```python
from build123d import *

# Parameters (mm, degrees)
SKETCH1_W                   = 203.2
SKETCH1_H                   = 44.4627
CHAMFER1_SIZE               = 1.524
CUT_EXTRUDE2_START          = -88.9254
SKETCH2_W                   = 44.45
SKETCH2_H                   = 38.1
CUT_EXTRUDE2_DEPTH          = 177.8508
FILLET1_R                   = 6.35
CUT_EXTRUDE4_START          = 31.7627
SKETCH3_W                   = 47.752
SKETCH3_H                   = 44.45
CUT_EXTRUDE4_DEPTH          = 88.9254
FILLET2_R                   = 6.35
CUT_EXTRUDE6_START          = -101.6
SKETCH4_R                   = 18.0578125
CUT_EXTRUDE6_DEPTH          = 63.5
CUT_EXTRUDE8_START          = 101.6
SKETCH5_R                   = 6.7437
CUT_EXTRUDE8_DEPTH          = 95.25
CUT_EXTRUDE10_START         = 101.6
SKETCH6_R                   = 10.3124
CUT_EXTRUDE10_DEPTH         = 31.75
F_3_8_16_TAPPED_HOLE2_D     = 7.9375
F_3_8_16_TAPPED_HOLE2_DEPTH = 22.352
F_3_8_16_TAPPED_HOLE2_TIP   = 2.384665582


with BuildPart() as part:
    # Sketch1 → Revolve1 (revolve)
    with BuildSketch(Plane(origin=(0, 0, 0), x_dir=(1, 0, 0), z_dir=(0, 1, 0)), mode=Mode.PRIVATE) as revolve1_sk:
        with Locations((0, 22.23135)):
            Rectangle(SKETCH1_W, SKETCH1_H)
    revolve(revolve1_sk.sketch.rotate(Axis((-127, 0, 0), (1, 0, 0)), 180), axis=Axis((-127, 0, 0), (1, 0, 0)))

    # Chamfer1
    chamfer1_edges = [part.edges().sort_by_distance(p)[0] for p in [
        (101.6, 0, -44.4627),
        (-101.6, 0, -44.4627),
    ]]
    chamfer(chamfer1_edges, length=CHAMFER1_SIZE)

    # Sketch2 → Cut-Extrude2 (cut)
    with BuildSketch(Plane(origin=(0, 0, 0), x_dir=(1, 0, 0), z_dir=(0, 1, 0)).offset(CUT_EXTRUDE2_START)):
        with Locations((-9.525, 0)):
            Rectangle(SKETCH2_W, SKETCH2_H)
    extrude(amount=CUT_EXTRUDE2_DEPTH, mode=Mode.SUBTRACT)

    # Fillet1
    fillet1_edges = [part.edges().sort_by_distance(p)[0] for p in [
        (-31.75, 0, -19.05),
        (-31.75, 0, 19.05),
        (12.7, 0, 19.05),
        (12.7, 0, -19.05),
    ]]
    fillet(fillet1_edges, radius=FILLET1_R)

    # Sketch3 → Cut-Extrude4 (cut)
    with BuildSketch(Plane(origin=(0, 0, 0), x_dir=(1, 0, 0), z_dir=(0, 1, 0)).offset(CUT_EXTRUDE4_START)):
        with Locations((-9.652, 0)):
            Rectangle(SKETCH3_W, SKETCH3_H)
    extrude(amount=CUT_EXTRUDE4_DEPTH, mode=Mode.SUBTRACT)

    # Fillet2
    fillet2_edges = [part.edges().sort_by_distance(p)[0] for p in [
        (-33.528, 35.136096599, -22.225),
        (-33.528, 35.136096599, 22.225),
        (14.224, 35.136096599, 22.225),
        (14.224, 35.136096599, -22.225),
    ]]
    fillet(fillet2_edges, radius=FILLET2_R)

    # Sketch4 → Cut-Extrude6 (cut)
    with BuildSketch(Plane(origin=(0, 0, 0), x_dir=(0, 0, -1), z_dir=(1, 0, 0)).offset(CUT_EXTRUDE6_START)):
        Circle(SKETCH4_R)
    extrude(amount=CUT_EXTRUDE6_DEPTH, mode=Mode.SUBTRACT)

    # Sketch5 → Cut-Extrude8 (cut)
    with BuildSketch(Plane(origin=(0, 0, 0), x_dir=(0, 0, -1), z_dir=(1, 0, 0)).offset(CUT_EXTRUDE8_START)):
        Circle(SKETCH5_R)
    extrude(amount=-CUT_EXTRUDE8_DEPTH, mode=Mode.SUBTRACT)

    # Sketch6 → Cut-Extrude10 (cut)
    with BuildSketch(Plane(origin=(0, 0, 0), x_dir=(0, 0, -1), z_dir=(1, 0, 0)).offset(CUT_EXTRUDE10_START)):
        Circle(SKETCH6_R)
    extrude(amount=-CUT_EXTRUDE10_DEPTH, mode=Mode.SUBTRACT)

    # 3/8-16 Tapped Hole2
    with Locations(Plane(origin=(101.6, 0, 0), x_dir=(0, 0, -1), z_dir=(1, 0, 0))):
        with Locations((-22.4536, -22.4536), (22.4536, -22.4536), (-22.4536, 22.4536), (22.4536, 22.4536)):
            Hole(F_3_8_16_TAPPED_HOLE2_D / 2, depth=F_3_8_16_TAPPED_HOLE2_DEPTH)
            with Locations((0, 0, -(F_3_8_16_TAPPED_HOLE2_DEPTH + F_3_8_16_TAPPED_HOLE2_TIP / 2))):  # 118° drill point
                Cone(0, F_3_8_16_TAPPED_HOLE2_D / 2, F_3_8_16_TAPPED_HOLE2_TIP, mode=Mode.SUBTRACT)


solid = part.part
```
Work out the finished part from the listing and answer in its coordinate system (mm). A direction names the side the tool comes from. Give positions to 0.01 mm unless a question says otherwise; leave off trailing zeros. Loops run counter-clockwise (first coordinate to the right, second up) from the corner with the lowest first, then second, coordinate; pieces in that order, holes last. Notation, with made-up numbers: (87.5, -9.5) - (94.5, -9.5) arc R28 cw to (94.5, 24.5) - close; hole circle Ø1 at (-10, -38). An arc over 180 degrees is marked (long way). One line per question, with ' | ' between items.
(1) Each of these flat-tipped pins is pushed along its axis until it touches: pin 1 Ø6 at (x, y) = (-32, -32.5) entering from +Z; pin 2 Ø7.5 at (x, y) = (-8, 33.5) entering from -Z; pin 3 Ø4 at (x, z) = (77, 27.5) entering from +Y. Where does it stop, or does it pass through?
Recorded:
pin 1: stops at z = 33.27 | pin 2: stops at z = -33.04 | pin 3: stops at y = 36.42
(2) The part is cut by section C-C (y = 0). Write down the section's boundary in (x, z).
Recorded:
outline: (-101.6, -42.94) - (-100.08, -44.46) - (100.08, -44.46) - (101.6, -42.94) - (101.6, -10.31) - (69.85, -10.31) - (69.85, -6.74) - (12.7, -6.74) - (12.7, -12.7) arc R6.35 cw to (6.35, -19.05) - (-25.4, -19.05) arc R6.35 cw to (-31.75, -12.7) - (-31.75, 12.7) arc R6.35 cw to (-25.4, 19.05) - (6.35, 19.05) arc R6.35 cw to (12.7, 12.7) - (12.7, 6.74) - (69.85, 6.74) - (69.85, 10.31) - (101.6, 10.31) - (101.6, 42.94) - (100.08, 44.46) - (-100.08, 44.46) - (-101.6, 42.94) - (-101.6, 18.06) - (-38.1, 18.06) - (-38.1, -18.06) - (-101.6, -18.06) - close
(3) The part is cut by section B-B (x = 54). Write down the section's boundary in (y, z).
Recorded:
outline: circle Ø88.93 at (0, 0); hole circle Ø13.49 at (0, 0)
(4) Straight lines are drawn through the part: probe 1 along Z at (x, y) = (-71.5, -1); probe 2 along Y at (x, z) = (-61.5, 0); probe 3 along X at (y, z) = (3, -7). For each, find the intervals that lie inside material, in ascending order.
Recorded:
probe 1: z = -44.45 to -18.03, 18.03 to 44.45 | probe 2: y = -44.46 to -18.06, 18.06 to 44.46 | probe 3: x = -38.1 to -31.75, 12.7 to 69.85
(5) The part is cut by section A-A (z = 0). Write down the section's boundary in (x, y), then the cut area to 3 significant figures.
Recorded:
outline: (-101.6, -42.94) - (-100.08, -44.46) - (-31.75, -44.46) - (-31.75, 31.76) - (-33.53, 31.76) - (-33.53, 44.46) - (-100.08, 44.46) - (-101.6, 42.94) - (-101.6, 18.06) - (-38.1, 18.06) - (-38.1, -18.06) - (-101.6, -18.06) - close; (12.7, -44.46) - (100.08, -44.46) - (101.6, -42.94) - (101.6, -10.31) - (69.85, -10.31) - (69.85, -6.74) - (12.7, -6.74) - close; (12.7, 6.74) - (69.85, 6.74) - (69.85, 10.31) - (101.6, 10.31) - (101.6, 42.94) - (100.08, 44.46) - (14.22, 44.46) - (14.22, 31.76) - (12.7, 31.76) - close | area: 10,400 mm²
(6) A tool of negligible diameter and unlimited length cuts with its end or side. For faces 4 (the face through (12.7, -7, 0)), 5 (the face through (85.95, 8.7, -5.54)), 6 (the face through (-70.29, -17.63, 3.91)), from which of +Z, -Z, +X, -X, +Y, -Y can it reach the whole face along a straight path? Write none if from no direction.
Recorded:
face 4: +Y, -Y | face 5: +X | face 6: -X
(7) The mould has two halves that part along X. Classify faces 1 (the face through (10.89, -4.9, 17.14)), 2 (the face through (41.675, -6.583, 1.462)), 3 (the face through (77.28, -21.77, -22.36)): +X half, -X half, draft (parallel to the pull), parting line (faces both ways), or undercut.
Recorded:
face 1: undercut | face 2: draft | face 3: +X half
